```python
from build123d import *

# Parameters (mm, degrees)
BOSS_EXTRUDE1_DEPTH = 35
BOSS_EXTRUDE2_DEPTH = 50
BOSS_EXTRUDE4_DEPTH = 4
SKETCH4_R           = 25
SKETCH4_R_2         = 12.5
BOSS_EXTRUDE5_DEPTH = 15


with BuildPart() as part:
    # Sketch1 → Boss-Extrude1 (new body)
    with BuildSketch(Plane(origin=(0, 0, 0), x_dir=(1, 0, 0), z_dir=(0, 1, 0))):
        with BuildLine():
            Line((-15.658362989, 25), (34.341637011, 25))
            ThreePointArc((34.341637011, 25), (59.341637011, 0), (34.341637011, -25))
            Line((34.341637011, -25), (-15.658362989, -25))
            ThreePointArc((-15.658362989, -25), (-40.658362989, 0), (-15.658362989, 25))
        make_face()
        with BuildLine():
            Line((-15.658362989, 10), (34.341637011, 10))
            ThreePointArc((34.341637011, 10), (44.341637011, 0), (34.341637011, -10))
            Line((34.341637011, -10), (-15.658362989, -10))
            ThreePointArc((-15.658362989, -10), (-25.658362989, 0), (-15.658362989, 10))
        make_face(mode=Mode.SUBTRACT)
    extrude(amount=-BOSS_EXTRUDE1_DEPTH)

    # Sketch2 → Boss-Extrude2 (add)
    with BuildSketch(Plane.XY.offset(25)):
        Polygon((59.341637011, -12.5), (34.341637011, -12.5), (34.341637011, -22.5), (59.341637011, -22.5), (149.341637011, -22.5), (149.341637011, -12.5), align=None)
    extrude(amount=-BOSS_EXTRUDE2_DEPTH)

    # Sketch3 → Boss-Extrude4 (add, symmetric)
    with BuildSketch(Plane.XY):
        with BuildLine():
            Line((58.524856224, -12.5), (59.341637011, -12.5))
            Line((59.341637011, -12.5), (149.341637011, -12.5))
            Line((149.341637011, -12.5), (149.341637011, 43))
            ThreePointArc((149.341637011, 43), (124.341637011, 18), (99.341637011, 43))
            Line((99.341637011, 43), (99.341637011, 11.044665925))
            ThreePointArc((99.341637011, 11.044665925), (93.33790357, -0.068272059), (81.509886267, -4.5))
            Line((81.509886267, -4.5), (58.524856224, -4.5))
            Line((58.524856224, -4.5), (58.524856224, -12.5))
        make_face()
    extrude(amount=BOSS_EXTRUDE4_DEPTH, both=True)

    # Sketch4 → Boss-Extrude5 (add, symmetric)
    with BuildSketch(Plane.XY):
        with Locations((124.341637011, 43)):
            Circle(SKETCH4_R)
        with Locations((124.341637011, 43)):
            Circle(SKETCH4_R_2, mode=Mode.SUBTRACT)
    extrude(amount=BOSS_EXTRUDE5_DEPTH, both=True)


solid = part.part
```
The listing builds one solid part. Answer for the finished solid, in the listing's coordinates (mm). A direction names the side the tool comes from. Coordinates: 2 decimals unless noted, no trailing zeros. Write each loop counter-clockwise with the first axis right and the second up, starting at its lowest first coordinate (ties: lowest second). Pieces come first, ordered by that corner, then holes. Notation, with made-up numbers: (-13, 32.5) - (-2, 32.5) arc R14 ccw to (-2, 54.5) - close; hole circle Ø3 at (84.25, -17.5). An arc over 180 degrees is marked (long way). One line per item, written item: value.
1) Consider line 1 along Z through (x, y) = (-10.5, -17.5); line 2 along Z through (x, y) = (83, -6.5); line 3 along Y through (x, z) = (5, 22.5). Determine where each line is inside the solid, lowest interval first. Write a range as from..to.
Geometry check:
line 1: z = -25..-10, 10..25
line 2: z = -4..4
line 3: y = -35..0
2) Find section C-C (x = 16.5). Give the vertices of the cut face in (y, z).
Geometry check:
outline: (-35, -25) - (0, -25) - (0, -10) - (-35, -10) - close; (-35, 10) - (0, 10) - (0, 25) - (-35, 25) - close
3) A tool of negligible diameter and unlimited length cuts with its end or side. For faces 4 (the flat face through (113, 49, -15)), 5 (the flat face through (113, 49, 15)), 6 (the flat face through (105, -12.5, 15)), 7 (the cylindrical face through (93.47, 0.05, 0.06)), 8 (the cylindrical face through (44.34, -28.66, -0.22)), from which of +Z, -Z, +X, -X, +Y, -Y can it reach the whole face along a straight path? Write none if from no direction.
Geometry check:
face 4: -Z, +X, -X, +Y
face 5: +Z, +X, -X, +Y
face 6: +Z, +X
face 7: +Z, -Z, +Y
face 8: -Y
4) Find section D-D (z = -12). Give the vertices of the cut face in (x, y).
Geometry check:
outline: (-37.59, -35) - (56.27, -35) - (56.27, -22.5) - (149.34, -22.5) - (149.34, -12.5) - (56.27, -12.5) - (56.27, 0) - (-37.59, 0) - close; circle Ø50 at (124.34, 43); hole circle Ø25 at (124.34, 43)
5) Each of these flat-tipped pins is pushed along its axis until it touches: pin 1 Ø10.5 at (x, z) = (65, 19) entering from +Y; pin 2 Ø15 at (x, y) = (117.5, 31) entering from -Z; pin 3 Ø11 at (y, z) = (-16, -3.5) entering from -X. Where does it stop, or does it pass through?
Geometry check:
pin 1: stops at y = -12.5
pin 2: stops at z = -15
pin 3: stops at x = -40.66
6) Find section B-B (y = -2). Give the vertices of the cut face in (x, z).
Geometry check:
outline: (-15.66, -25) - (34.34, -25) arc R25 ccw to (34.34, 25) - (-15.66, 25) arc R25 ccw to start; (90.66, -4) - (149.34, -4) - (149.34, 4) - (90.66, 4) - close; hole (-15.66, -10) - (34.34, -10) arc R10 ccw to (34.34, 10) - (-15.66, 10) arc R10 ccw to start
7) For a pull along Y with two mould halves and no side action, classify faces 1 (the flat face through (99.342, 27, 0)), 2 (the flat face through (114, 3, -4)), 3 (the flat face through (10, -35, 11)) as pulls with the +Y half, pulls with the -Y half, needs draft (parallel to the pull), parting line crosses it, or undercut.
Geometry check:
face 1: needs draft
face 2: undercut
face 3: pulls with the -Y half
8) Find section A-A (z = 0). Give the vertices of the cut face in (x, y).
Geometry check:
outline: (-40.66, -35) - (-25.66, -35) - (-25.66, 0) - (-40.66, 0) - close; (34.34, -22.5) - (44.34, -22.5) - (44.34, -35) - (59.34, -35) - (59.34, -22.5) - (149.34, -22.5) - (149.34, 43) arc R25 ccw to (99.34, 43) - (99.34, 11.04) arc R18 cw to (81.51, -4.5) - (59.34, -4.5) - (59.34, 0) - (44.34, 0) - (44.34, -12.5) - (34.34, -12.5) - close; hole circle Ø25 at (124.34, 43)
